Autodesk Inventor part; units mm, degrees
ref_plane "YZ Plane" through (0, 0, 0) normal (1, 0, 0) x (0, 1, 0)
ref_plane "XZ Plane" through (0, 0, 0) normal (0, 1, 0) x (-1, 0, 0)
ref_plane "XY Plane" through (0, 0, 0) normal (0, 0, 1) x (1, 0, 0)
sketch "Эскиз1" plane through (0, 0, 0) normal (1, 0, 0) x (0, 1, 0)
  line L0 (10, -2.5) -> (10, -5.75)
  line L1 (10, -5.75) -> (9, -5.75)
  line L2 (9, -5.75) -> (9, -3.75)
  line L3 (9, -3.75) -> (0, -3.75)
  line L4 (0, -3.75) -> (0, -2.5)
  line L5 (0, -2.5) -> (10, -2.5)
  line L6 (-2, 0) -> (12, 0)
  point P0 (0, 0)
  dimension "d0" = 2.5
  dimension "d1" = 3.75
  dimension "d2" = 1
  dimension "d3" = 10
  dimension "d4" = 5.75
revolve "Вращение1" add sketch "Эскиз1" angle 360 about axis through (0, -10, 0) along (0, 1, 0)
chamfer "Фаска1" distance 0.25 angle 45 3 edges at (0, 10, 2.5) (0, 0, 2.5) (0, 0, 3.75)
chamfer "Фаска2" distance 0.25 angle 45 2 edges at (0, 9, 5.75) (0, 10, 5.75)
properties part number "sleeve" material "Алюминий 6061-AHC"
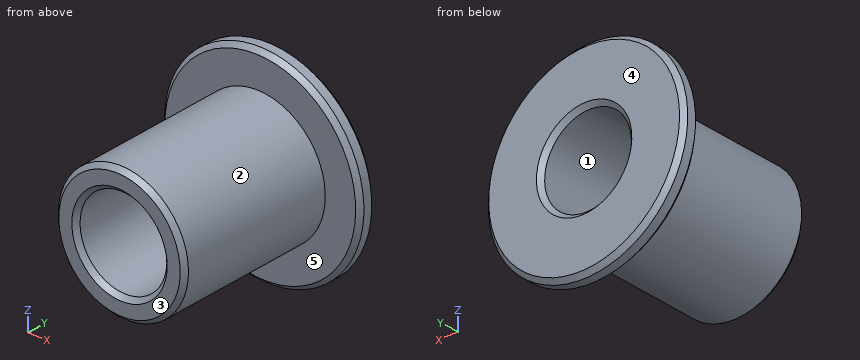
Check sheet for the modelled part. Datum: model origin and axes. Units: mm. Face numbers are marked on the shaded views. A direction names the side the tool comes from. Round coordinates to 2 decimals unless told otherwise and drop trailing zeros. Write each loop counter-clockwise with the first axis right and the second up, starting at its lowest first coordinate (ties: lowest second). Pieces come first, ordered by that corner, then holes. Notation, with made-up numbers: (10.5, 50.5) -> (27.5, 50.5) arc R19 ccw to (27.5, 61.5) -> close; hole circle Ø9 at (56, -18). An arc over 180 degrees is marked (long way). One line per question, with ' | ' between items. Start each with the question number.
1. Sectioned sample at A-A, the plane z = 0. Record the cut outline in (x, y), then the cut area to 3 significant figures.
2. Sectioned sample at C-C, the plane y = 4.75. Record the cut outline in (x, z).
3. Sectioned sample at B-B, the plane x = 0. Record the cut outline in (y, z), then the cut area to 3 significant figures.
4. Depth check by flat-ended pin: pin 1 (5.5 mm diameter, centred on x = 1, z = 2, fed in from -Y); pin 2 (1.5 mm diameter, centred on x = -4, y = 1.5, fed in from +Z); pin 3 (3 mm diameter, centred on y = 3, z = -1, fed in from +X). Enter the tip coordinate at first touch or a pass-through.
5. Scan lines: line 1 along Z through (x, y) = (0, 4.25); line 2 along Y through (x, z) = (-4.5, 1.5). Record each from-to range of solid material in increasing order. Write a range as from..to.
6. Set-up check for the marked faces 4 and 5: record each of +Z, -Z, +X, -X, +Y, -Y from which the full face is reachable in a straight line by a thin tool's end or side.
7. Release check for a two-part mould opening along Z. For the marked faces 1, 2 and 3 record: +Z half, -Z half, draft (parallel to the pull), parting line (faces both ways), or undercut.
Taken from the geometry:
1) outline: (-5.75, 9.25) -> (-5.5, 9) -> (-3.75, 9) -> (-3.75, 0.25) -> (-3.5, 0) -> (-2.75, 0) -> (-2.5, 0.25) -> (-2.5, 9.75) -> (-2.75, 10) -> (-5.5, 10) -> (-5.75, 9.75) -> close; (2.5, 0.25) -> (2.75, 0) -> (3.5, 0) -> (3.75, 0.25) -> (3.75, 9) -> (5.5, 9) -> (5.75, 9.25) -> (5.75, 9.75) -> (5.5, 10) -> (2.75, 10) -> (2.5, 9.75) -> close | area: 28.7 mm^2
2) outline: circle Ø7.5 at (0, 0); hole circle Ø5 at (0, 0)
3) outline: (0, -3.5) -> (0.25, -3.75) -> (9, -3.75) -> (9, -5.5) -> (9.25, -5.75) -> (9.75, -5.75) -> (10, -5.5) -> (10, -2.75) -> (9.75, -2.5) -> (0.25, -2.5) -> (0, -2.75) -> close; (0, 2.75) -> (0.25, 2.5) -> (9.75, 2.5) -> (10, 2.75) -> (10, 5.5) -> (9.75, 5.75) -> (9.25, 5.75) -> (9, 5.5) -> (9, 3.75) -> (0.25, 3.75) -> (0, 3.5) -> close | area: 28.7 mm^2
4) pin 1: stops at y = 0 | pin 2: stops at z = 1.87 | pin 3: stops at x = 3.75
5) line 1: z = -3.75..-2.5, 2.5..3.75 | line 2: y = 9..10
6) face 4: +Z, -Z, +X, -X, +Y | face 5: -Y
7) face 1: undercut | face 2: parting line | face 3: draft
